Part print with two shaded views. Sizes in mm from the minimum x, y, z corner. Coordinates: 2 decimals unless noted, no trailing zeros. Order: outer loops, then holes, each group sorted by start corner. A loop starts at its lowest first (then second) coordinate and runs counter-clockwise, first axis right, second up. Notation, with made-up numbers: (84, 8) - (115, 8) arc R11 cw to (115, 22) - close; hole circle Ø2 at (8.25, -37). An arc over 180 degrees is marked (long way). Write each question's results on one line, items separated by ' | '. Start each with the question number.
Q1. Band-saw the part on C-C, the plane z = 19.5. Write the cut outline in (x, y), then the cut area to 3 significant figures.
Q2. Wall check: probe 1 along Y at (x, z) = (47.5, 8); probe 2 along Y at (x, z) = (24, 34.5); probe 3 along X at (y, z) = (12.5, 33) (1 decimal). Give the ranges that are in metal, low to high.
Q3. Band-saw the part on D-D, the plane x = 52.5. Write the cut outline in (y, z), then the cut area to 3 significant figures.
Q4. Pull direction X, two halves, no side cores. Call the marked faces 1, 2, 3 and 4: released by +X, released by -X, zero draft, split by the parting line, or undercut.
Q5. Band-saw the part on B-B, the plane x = 24. Write the cut outline in (y, z).
Q6. Band-saw the part on A-A, the plane y = 33. Write the cut outline in (x, z), then the cut area to 3 significant figures.
Q7. Pin check, flat tips, straight feed: P1, Ø6.5, axis at x = 23, y = 8, coming from the +Z side; P2, Ø5, axis at y = 58, z = 8, coming from the -X side; P3, Ø7, axis at y = 8, z = 8, coming from the -X side; P4, Ø5, axis at x = 24, y = 58.5, coming from the +Z side. Stop position of each tip, or through.
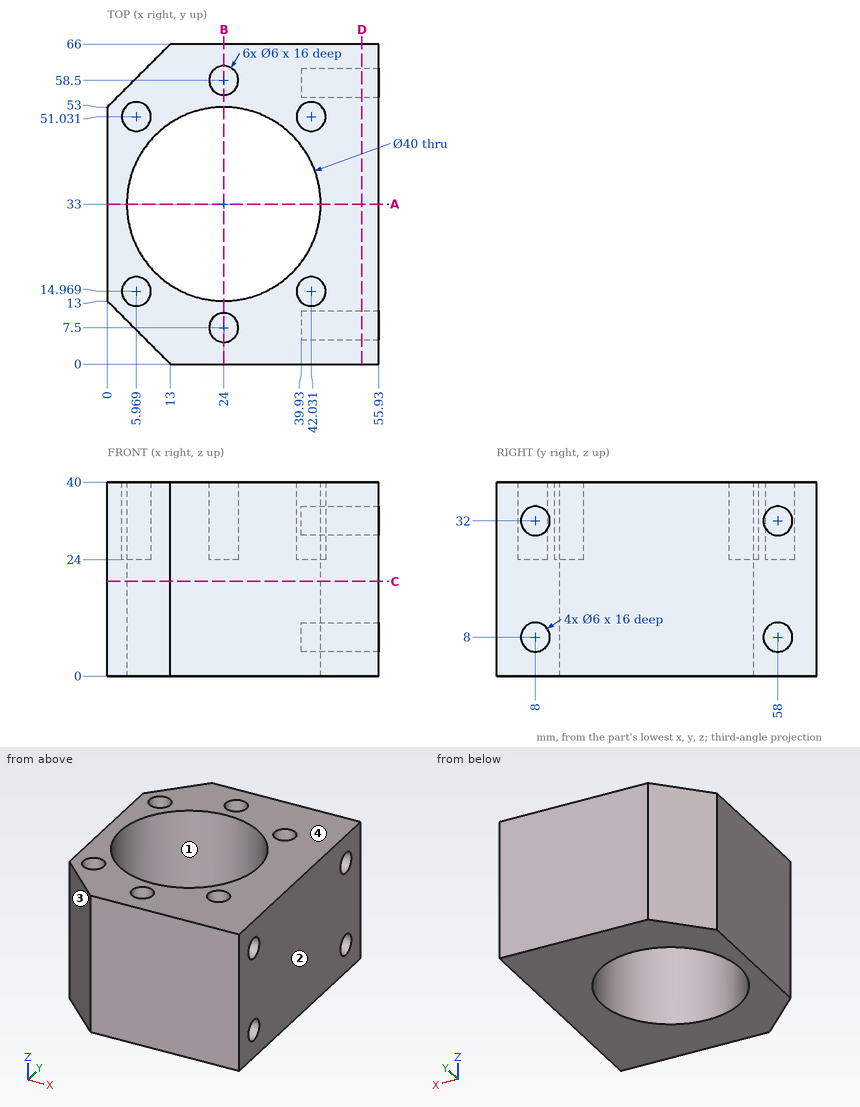
Results below:
1) outline: (0, 13) - (13, 0) - (55.93, 0) - (55.93, 66) - (13, 66) - (0, 53) - close; hole circle Ø40 at (24, 33) | area: 2,270 mm²
2) probe 1: y = 0 to 5, 11 to 55, 61 to 66 | probe 2: y = 0 to 4.5, 10.5 to 13, 53 to 55.5, 61.5 to 66 | probe 3: x = 0.5 to 4.3, 7.7 to 40.3, 43.7 to 55.9
3) outline: (0, 0) - (66, 0) - (66, 40) - (0, 40) - close; hole circle Ø6 at (8, 8); hole circle Ø6 at (8, 32); hole circle Ø6 at (58, 8); hole circle Ø6 at (58, 32) | area: 2,530 mm²
4) face 1: undercut | face 2: released by +X | face 3: released by -X | face 4: zero draft
5) outline: (0, 0) - (13, 0) - (13, 40) - (10.5, 40) - (10.5, 24) - (4.5, 24) - (4.5, 40) - (0, 40) - close; (53, 0) - (66, 0) - (66, 40) - (61.5, 40) - (61.5, 24) - (55.5, 24) - (55.5, 40) - (53, 40) - close
6) outline: (0, 0) - (4, 0) - (4, 40) - (0, 40) - close; (44, 0) - (55.93, 0) - (55.93, 40) - (44, 40) - close | area: 637 mm²
7) P1: stops at z = 40 | P2: stops at x = 2.5 | P3: stops at x = 1.5 | P4: stops at z = 24
